from build123d import *

# Parameters (mm, degrees)
BOSS_EXTRUDE1_DEPTH = 6.35


with BuildPart() as part:
    # Sketch1 → Boss-Extrude1 (new body)
    with BuildSketch(Plane(origin=(0, 0, 0), x_dir=(1, 0, 0), z_dir=(0, 1, 0))):
        with BuildLine():
            Line((-99.020583087, -242.427582229), (-99.020583087, -374.65))
            ThreePointArc((-99.020583087, -374.65), (-89.495583087, -384.175), (-79.970583087, -374.65))
            Line((-79.970583087, -374.65), (-79.970583087, -245.266880288))
            ThreePointArc((-79.970583087, -245.266880288), (-78.028039526, -219.05629054), (-72.242855135, -193.418425341))
            Line((-72.242855135, -193.418425341), (-69.161727013, -183.311770075))
            ThreePointArc((-69.161727013, -183.311770075), (-36.664014716, -108.894116093), (12.050429612, -43.924958467))
            ThreePointArc((12.050429612, -43.924958467), (12.501856954, -40.160483954), (9.02530478, -38.647658789))
            ThreePointArc((9.02530478, -38.647658789), (-15.385960803, -36.583737732), (-33.934614128, -20.580078236))
            ThreePointArc((-33.934614128, -20.580078236), (-37.044039814, -19.076108136), (-39.686388117, -21.300619228))
            Line((-39.686388117, -21.300619228), (-91.292855135, -190.579127282))
            ThreePointArc((-91.292855135, -190.579127282), (-97.078039526, -216.216992482), (-99.020583087, -242.427582229))
        make_face()
    extrude(amount=BOSS_EXTRUDE1_DEPTH)


solid = part.part
Input: part model. Units: mm. Frame: model coordinates. A direction names the side the tool comes from. Round coordinates to 2 decimals unless told otherwise and drop trailing zeros. Write each loop counter-clockwise with the first axis right and the second up, starting at its lowest first coordinate (ties: lowest second). Pieces come first, ordered by that corner, then holes.
1) Contact query for flat-ended pins moving along their axis: P1, Ø2, axis at y = 1, z = 151, coming from the -X side; P2, Ø3, axis at y = 4, z = 288, coming from the +X side; P3, Ø3, axis at y = 2.5, z = 127, coming from the +X side. Output: stop coordinate, or through.
2) Ray query, L1, parallel to X at y = 3.5, z = 332.5; L2, parallel to Z at x = -31, y = 5.5; L3, parallel to Z at x = -8, y = 3.5 (3 decimals). Return the intervals inside material, ascending.
3) Cut plane B-B (x = -44.5). Return the cut outline in (y, z), then the cut area to 3 significant figures.
4) Reachability of faces 1 (the cylindrical face through (-97.023, 3.131, 215.853)), 2 (the flat face through (-79.971, 3, 311)) from +Z, -Z, +X, -X, +Y, -Y: full face, straight path, thin tool, end or side. Return the list, or none.
5) Cut plane C-C (z = 138). Return the cut outline in (x, y).
Geometry says:
1. P1: stops at x = -79.53
1. P2: stops at x = -79.97
1. P3: stops at x = -45.75
2. L1: x = -99.02 to -79.97
2. L2: z = 24.78 to 99.51
2. L3: z = 38.873 to 66.985
3. outline: (0, 37.09) - (6.35, 37.09) - (6.35, 123.09) - (0, 123.09) - close
3. area: 546 mm2
4. face 1: -Z, -X, +Y, -Y
4. face 2: +Z, +X, +Y, -Y
5. outline: (-75.26, 0) - (-51.85, 0) - (-51.85, 6.35) - (-75.26, 6.35) - close
